Model file for the job. Use its own axes, mm. A direction names the side the tool comes from. Give positions to 0.01 mm unless a question says otherwise; leave off trailing zeros. Loops run counter-clockwise (first coordinate to the right, second up) from the corner with the lowest first, then second, coordinate; pieces in that order, holes last. Notation, with made-up numbers: M 54.25,-26 L 104.25,-26 A27 ccw 104.25,11 Z; hole C -28,63.5 d8. An arc over 180 degrees is marked long. Use CSV: the item, a comma, the result in double quotes. Start each with the question number.
(1) Slice it at B-B on x = -46. List the corners of the cut face in (y, z), and give its area (3 significant figures).
(2) Slice it at C-C on z = -7.5. List the corners of the cut face in (x, y).
(3) Slice it at D-D on x = -36.5. List the corners of the cut face in (y, z).
(4) Slice it at A-A on y = 9. State how many separate pieces and enclosed holes the cut face has, and give its area (3 significant figures).
(5) Wall check: line 1 along X through (y, z) = (5, 44); line 2 along X through (y, z) = (4.25, 13); line 3 along X through (y, z) = (2.25, 31). Give the ranges that are in metal, low to high. Write a range as from..to.
(6) Two-plate mould, pull along Z, no slides. Class faces 3 (the face through (-18.207, 4.93, 52.732)), 4 (the face through (-11, 10, 35)), 5 (the face through (-1.793, 4.93, -0.77)), 6 (the face through (16.722, 4.93, 33.546)): pulls with the +Z half, pulls with the -Z half, needs draft (parallel to the pull), parting line crosses it, or undercut.
(7) Tool access for faces 1 (the face through (-40.28, 4.93, 24.33)), 2 (the face through (-15, 5, 26)): list every direction of +Z, -Z, +X, -X, +Y, -Y with a clear straight run to the whole face (end or side of a thin tool).
(8) Flat gauge pins, fed straight in: P1, Ø5, axis at x = -10.5, y = 5.5, coming from the -Z side; P2, Ø8, axis at x = -35, z = 60.622, coming from the +Y side; P3, Ø5, axis at x = -17.5, y = 2.5, coming from the -Z side; P4, Ø2, axis at y = 4, z = 14, coming from the -X side. Where does each tip first touch, or does it go through?
```python
from build123d import *

# Parameters (mm, degrees)
SKETCH1_R           = 5.05
BOSS_EXTRUDE1_DEPTH = 10
FILLET1_R           = 1


with BuildPart() as part:
    # Sketch1 → Boss-Extrude1 (new body)
    # profile 1 of 14: a face of its own
    with BuildSketch(Plane(origin=(0, 0, 0), x_dir=(1, 0, 0), z_dir=(0, 1, 0))):
        Polygon((2.667006003, -23.808109615), (-5, -18.496177846), (-5, -33.48105), (-14.97816514, -33.48105), (-11.765381702, -35.706962749), (-4.621337732, -33.907173957), align=None)
    # profile 2 of 14: a face of its own
    with BuildSketch(Plane(origin=(0, 0, 0), x_dir=(1, 0, 0), z_dir=(0, 1, 0))):
        Polygon((-5.02183486, -18.48105), (-8.234724145, -16.255063917), (-15.378926884, -18.054892707), (-22.667198451, -28.153857051), (-15, -33.465922154), (-15, -18.48105), align=None)
    # profile 3 of 14: a face of its own
    with BuildSketch(Plane(origin=(0, 0, 0), x_dir=(1, 0, 0), z_dir=(0, 1, 0))):
        Polygon((-8.234724145, -16.255063917), (-12.131573163, -13.555210012), (-15.378926884, -18.054892707), align=None)
    # profile 4 of 14: a face of its own
    with BuildSketch(Plane(origin=(0, 0, 0), x_dir=(1, 0, 0), z_dir=(0, 1, 0))):
        Polygon((-7.868619286, -38.406756654), (-4.621337732, -33.907173957), (-11.765381702, -35.706962749), align=None)
    # profile 5 of 14: a face of its own
    with BuildSketch(Plane(origin=(0, 0, 0), x_dir=(1, 0, 0), z_dir=(0, 1, 0))):
        Polygon((-15, -33.465922154), (-22.667198451, -28.153857051), (-31.751988504, -40.742160048), (-11.765381702, -35.706962749), (-14.97816514, -33.48105), (-15, -33.48105), align=None)
    # profile 6 of 14: a face of its own
    with BuildSketch(Plane(origin=(0, 0, 0), x_dir=(1, 0, 0), z_dir=(0, 1, 0))):
        Polygon((-22.667198451, -28.153857051), (-15.378926884, -18.054892707), (-31.413179434, -22.094379046), align=None)
    # profile 7 of 14: a face of its own
    with BuildSketch(Plane(origin=(0, 0, 0), x_dir=(1, 0, 0), z_dir=(0, 1, 0))):
        Polygon((11.413073587, -29.86764762), (2.667006003, -23.808109615), (-4.621337732, -33.907173957), align=None)
    # profile 8 of 14: a face of its own
    with BuildSketch(Plane(origin=(0, 0, 0), x_dir=(1, 0, 0), z_dir=(0, 1, 0))):
        Polygon((11.751723888, -11.219906616), (-8.234724145, -16.255063917), (-5.02183486, -18.48105), (-5, -18.48105), (-5, -18.496177846), (2.667006003, -23.808109615), align=None)
    # profile 9 of 14: a face of its own
    with BuildSketch(Plane(origin=(0, 0, 0), x_dir=(1, 0, 0), z_dir=(0, 1, 0))):
        with BuildLine():
            Line((7.702026656, 13.927138243), (-12.131573163, -13.555210012))
            Line((-12.131573163, -13.555210012), (-8.234724145, -16.255063917))
            Line((-8.234724145, -16.255063917), (11.751723888, -11.219906616))
            Line((11.751723888, -11.219906616), (22.297973344, 3.393461757))
            ThreePointArc((22.297973344, 3.393461757), (20.266838243, 15.958273344), (7.702026656, 13.927138243))
        make_face()
        with Locations(Location((15, 8.6603, 0), (0, 0, 270))):
            Circle(SKETCH1_R, mode=Mode.SUBTRACT)
    # profile 10 of 14: a face of its own
    with BuildSketch(Plane(origin=(0, 0, 0), x_dir=(1, 0, 0), z_dir=(0, 1, 0))):
        with BuildLine():
            Line((-12.131573163, -13.555210012), (-29.874498452, -1.262379084))
            ThreePointArc((-29.874498452, -1.262379084), (-42.397920916, -3.534798452), (-40.125501548, -16.058220916))
            Line((-40.125501548, -16.058220916), (-31.413179434, -22.094379046))
            Line((-31.413179434, -22.094379046), (-15.378926884, -18.054892707))
            Line((-15.378926884, -18.054892707), (-12.131573163, -13.555210012))
        make_face()
        with Locations(Location((-35, -8.6603, 0), (0, 0, 270))):
            Circle(SKETCH1_R, mode=Mode.SUBTRACT)
    # profile 11 of 14: a face of its own
    with BuildSketch(Plane(origin=(0, 0, 0), x_dir=(1, 0, 0), z_dir=(0, 1, 0))):
        with BuildLine():
            Line((22.801341803, -8.43619216), (11.751723888, -11.219906616))
            Line((11.751723888, -11.219906616), (2.667006003, -23.808109615))
            Line((2.667006003, -23.808109615), (11.413073587, -29.86764762))
            Line((11.413073587, -29.86764762), (27.198658197, -25.89080784))
            ThreePointArc((27.198658197, -25.89080784), (33.72730784, -14.964841803), (22.801341803, -8.43619216))
        make_face()
        with Locations(Location((25, -17.1635, 0), (0, 0, 270))):
            Circle(SKETCH1_R, mode=Mode.SUBTRACT)
    # profile 12 of 14: a face of its own
    with BuildSketch(Plane(origin=(0, 0, 0), x_dir=(1, 0, 0), z_dir=(0, 1, 0))):
        with BuildLine():
            Line((20.125501548, -35.903879084), (11.413073587, -29.86764762))
            Line((11.413073587, -29.86764762), (-4.621337732, -33.907173957))
            Line((-4.621337732, -33.907173957), (-7.868619286, -38.406756654))
            Line((-7.868619286, -38.406756654), (9.874498452, -50.699720916))
            ThreePointArc((9.874498452, -50.699720916), (22.397920916, -48.427301548), (20.125501548, -35.903879084))
        make_face()
        with Locations(Location((15, -43.3018, 0), (0, 0, 270))):
            Circle(SKETCH1_R, mode=Mode.SUBTRACT)
    # profile 13 of 14: a face of its own
    with BuildSketch(Plane(origin=(0, 0, 0), x_dir=(1, 0, 0), z_dir=(0, 1, 0))):
        with BuildLine():
            Line((-11.765381702, -35.706962749), (-31.751988504, -40.742160048))
            Line((-31.751988504, -40.742160048), (-42.297973344, -55.355161757))
            ThreePointArc((-42.297973344, -55.355161757), (-40.266838243, -67.919973344), (-27.702026656, -65.888838243))
            Line((-27.702026656, -65.888838243), (-7.868619286, -38.406756654))
            Line((-7.868619286, -38.406756654), (-11.765381702, -35.706962749))
        make_face()
        with Locations(Location((-35, -60.622, 0), (0, 0, 270))):
            Circle(SKETCH1_R, mode=Mode.SUBTRACT)
    # profile 14 of 14: a face of its own
    with BuildSketch(Plane(origin=(0, 0, 0), x_dir=(1, 0, 0), z_dir=(0, 1, 0))):
        with BuildLine():
            Line((-22.667198451, -28.153857051), (-31.413179434, -22.094379046))
            Line((-31.413179434, -22.094379046), (-47.198658197, -26.07119216))
            ThreePointArc((-47.198658197, -26.07119216), (-53.72730784, -36.997158197), (-42.801341803, -43.52580784))
            Line((-42.801341803, -43.52580784), (-31.751988504, -40.742160048))
            Line((-31.751988504, -40.742160048), (-22.667198451, -28.153857051))
        make_face()
        with Locations(Location((-45, -34.7985, 0), (0, 0, 270))):
            Circle(SKETCH1_R, mode=Mode.SUBTRACT)
    extrude(amount=BOSS_EXTRUDE1_DEPTH)

    # Fillet1
    fillet1_edges = [part.edges().sort_by_distance(p)[0] for p in [
        (-31.751988504, 5, 40.742160048),
        (-31.413179434, 5, 22.094379046),
        (-12.131573163, 5, 13.555210012),
        (11.751723888, 5, 11.219906616),
        (11.413073587, 5, 29.86764762),
        (-7.868619286, 5, 38.406756654),
    ]]
    fillet(fillet1_edges, radius=FILLET1_R)


solid = part.part
```
Reply:
1,outline,"M 0,25.77 L 10,25.77 L 10,29.85 L 0,29.85 Z; M 0,39.75 L 10,39.75 L 10,43.74 L 0,43.74 Z"
1,area,"80.7 mm^2"
2,outline,"M 3.06,0 L 10.09,0 L 10.09,10 L 3.06,10 Z; M 19.91,0 L 23.92,0 L 23.92,10 L 19.91,10 Z"
3,outline,"M 0,-0.21 L 10,-0.21 L 10,3.84 L 0,3.84 Z; M 0,13.48 L 10,13.48 L 10,18.57 L 0,18.57 Z; M 0,23.38 L 10,23.38 L 10,41.94 L 0,41.94 Z; M 0,47.32 L 10,47.32 L 10,55.8 L 0,55.8 Z; M 0,65.44 L 10,65.44 L 10,69.5 L 0,69.5 Z"
4,separate pieces,"1"
4,enclosed holes,"7"
4,area,"3,110 mm^2"
5,line 1,"x = -34.1..-11.91, 0.2..10, 20..23.97"
5,line 2,"x = -42.88..-37.58, -32.42..-12.93, -11.8..22.14, 27.86..32.98"
5,line 3,"x = -53.16..-48.33, -41.67..-15, -5..13.08"
6,face 3,"pulls with the +Z half"
6,face 4,"needs draft"
6,face 5,"pulls with the -Z half"
6,face 6,"undercut"
7,face 1,"-X, +Y, -Y"
7,face 2,"+Y, -Y"
8,P1,"stops at z = 7.83"
8,P2,"passes through"
8,P3,"stops at z = 8.1"
8,P4,"stops at x = -42.88"
